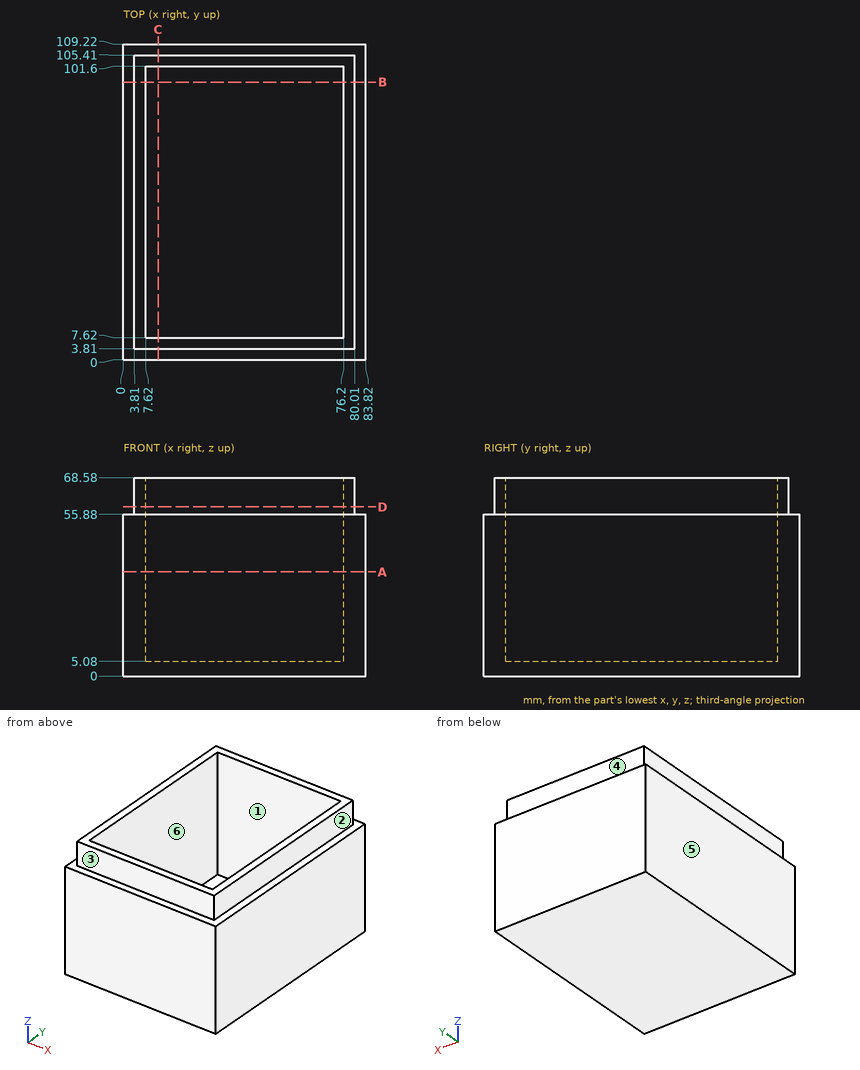
Design review of the part shown in the three views and the two pictorial views. Dimensions are in mm from the part's minimum x, y and z. A direction names the side the tool comes from. Give positions to 0.01 mm unless a question says otherwise; leave off trailing zeros. Loops run counter-clockwise (first coordinate to the right, second up) from the corner with the lowest first, then second, coordinate; pieces in that order, holes last. Notation, with made-up numbers: M 59.25,83.5 L 80.25,83.5 A16 ccw 80.25,93.5 Z; hole C 4,-1.5 d5. An arc over 180 degrees is marked long. Answer as a JSON object with one key per item and string values.
Item 1: We need section D-D (z = 58.5). State the section outline as (x, y) points.
Output values:
{"outline": "M 3.81,3.81 L 80.01,3.81 L 80.01,105.41 L 3.81,105.41 Z; hole M 7.62,7.62 L 76.2,7.62 L 76.2,101.6 L 7.62,101.6 Z"}
Item 2: We need section B-B (y = 96). State the section outline as (x, z) points, and give its area (3 significant figures).
Output values:
{"outline": "M 0,0 L 83.82,0 L 83.82,55.88 L 80.01,55.88 L 80.01,68.58 L 76.2,68.58 L 76.2,5.08 L 7.62,5.08 L 7.62,68.58 L 3.81,68.58 L 3.81,55.88 L 0,55.88 Z", "area": "1,300 mm2"}
Item 3: Wall thickness on line 1 along Y through (x, z) = (51.5, 62); line 2 along Y through (x, z) = (42.5, 37.5); line 3 along X through (y, z) = (8, 35): over which ranges is each line inside the solid? List them lowest first.
Output values:
{"line 1": "y = 3.81 to 7.62, 101.6 to 105.41", "line 2": "y = 0 to 7.62, 101.6 to 109.22", "line 3": "x = 0 to 7.62, 76.2 to 83.82"}
Item 4: We need section A-A (z = 36). State the section outline as (x, y) points.
Output values:
{"outline": "M 0,0 L 83.82,0 L 83.82,109.22 L 0,109.22 Z; hole M 7.62,7.62 L 76.2,7.62 L 76.2,101.6 L 7.62,101.6 Z"}
Item 5: Machinability: for the marked faces 1, 2 and 3, which of the approach directions +Z, -Z, +X, -X, +Y, -Y give a long, thin tool a straight path to every point of the face, cutting with its end or side? Answer none if there is none.
Output values:
{"face 1": "+Z", "face 2": "+Z, +X, +Y, -Y", "face 3": "+Z, +X, -X, -Y"}
Item 6: Mouldability with a two-part tool opening along X and no side actions: class the marked faces 4, 5 and 6 as pulls with the +X half, pulls with the -X half, needs draft (parallel to the pull), parting line crosses it, or undercut.
Output values:
{"face 4": "needs draft", "face 5": "pulls with the -X half", "face 6": "undercut"}
Item 7: We need section C-C (x = 12). State the section outline as (y, z) points, and give its area (3 significant figures).
Output values:
{"outline": "M 0,0 L 109.22,0 L 109.22,55.88 L 105.41,55.88 L 105.41,68.58 L 101.6,68.58 L 101.6,5.08 L 7.62,5.08 L 7.62,68.58 L 3.81,68.58 L 3.81,55.88 L 0,55.88 Z", "area": "1,430 mm2"}
Item 8: For P1, Ø10, axis at x = 41, z = 64, coming from the +Y side; P2, Ø1.5, axis at x = 63.5, z = 25.5, coming from the -Y side; P3, Ø20.5, axis at x = 56.5, y = 53, coming from the +Z side; P4, Ø10, axis at x = 54.5, z = 62.5, coming from the -Y side, all flat-tipped, find the tip position at first contact; note any pin that passes through.
Output values:
{"P1": "stops at y = 105.41", "P2": "stops at y = 0", "P3": "stops at z = 5.08", "P4": "stops at y = 3.81"}
